Geometry: see drawing. Coordinates: mm, zero at the bounding-box minimum. A direction names the side the tool comes from. Coordinates: 2 decimals unless noted, no trailing zeros. Write each loop counter-clockwise with the first axis right and the second up, starting at its lowest first coordinate (ties: lowest second). Pieces come first, ordered by that corner, then holes. Notation, with made-up numbers: (54, 87.5) - (70, 87.5) arc R21 cw to (70, 113.5) - close; hole circle Ø11 at (-6, -20.75). An arc over 180 degrees is marked (long way). One line per question, with ' | ' between items. Start each with the question number.
1) Draft query along Y for the marked faces 1, 2 and 3. Return one class per face: released by +Y, released by -Y, zero draft, split by the parting line, or undercut.
2) Line query: line 1 (Z direction, x = 16.2, y = 26.2); line 2 (Y direction, x = 9.35, z = 1.75); line 3 (Z direction, x = 17.75, y = 1.75). Output: solid intervals per line, ascending.
3) Section query D-D on z = 8. Return loops of the section in (x, y), and give its area (3 significant figures).
4) Section query A-A on y = 14.35. Return loops of the section in (x, z), and give its area (3 significant figures).
5) First-contact query: P1, Ø8, axis at x = 9.35, y = 14.35, coming from the +Z side. Flat tip, straight axial feed; report the tip coordinate or a pass-through.
6) Section query B-B on z = 0.75. Return loops of the section in (x, y), and give its area (3 significant figures).
7) Reachability of the marked faces 4 and 5 from +Z, -Z, +X, -X, +Y, -Y: full face, straight path, thin tool, end or side. Return the list, or none.
8) Section query C-C on x = 17.5. Return loops of the section in (y, z), and give its area (3 significant figures).
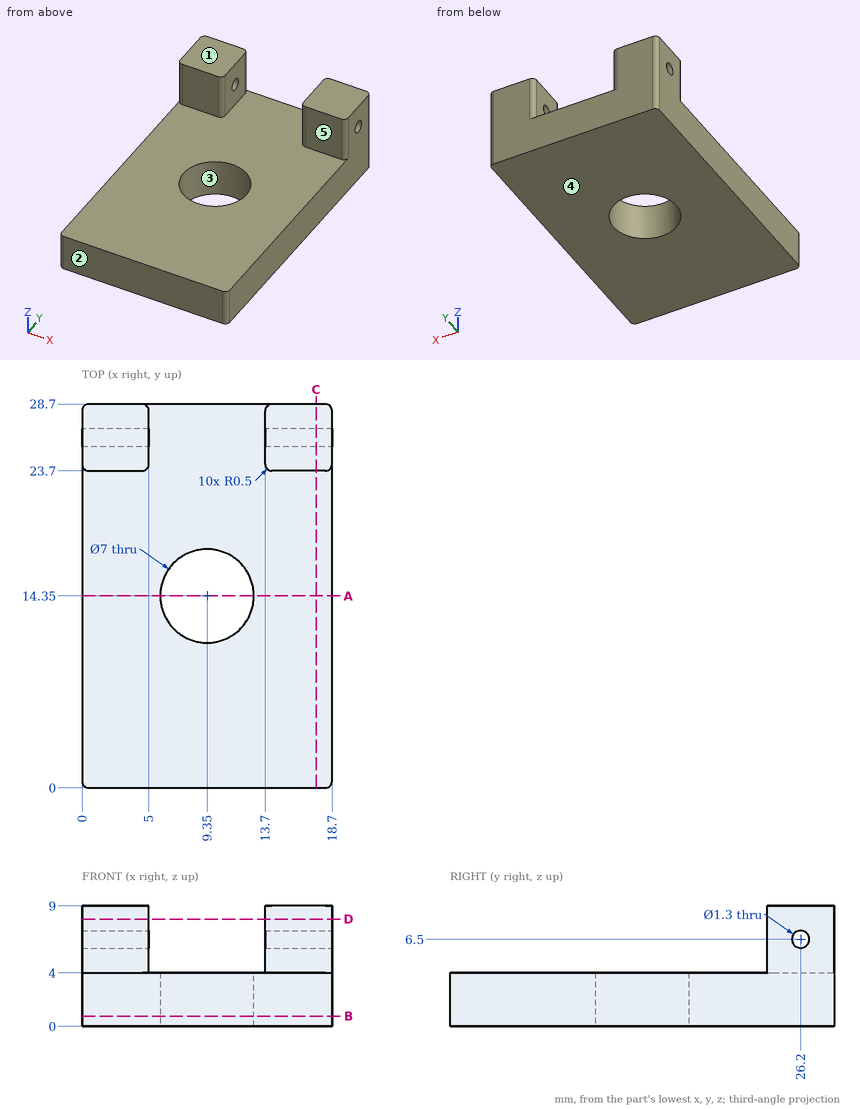
Answer key:
1) face 1: zero draft | face 2: released by -Y | face 3: undercut
2) line 1: 0 to 5.85, 7.15 to 9 | line 2: 0 to 10.85, 17.85 to 28.7 | line 3: 0 to 4
3) outline: (0, 24.2) arc R0.5 ccw to (0.5, 23.7) - (4.5, 23.7) arc R0.5 ccw to (5, 24.2) - (5, 28.2) arc R0.5 ccw to (4.5, 28.7) - (0.5, 28.7) arc R0.5 ccw to (0, 28.2) - close; (13.7, 24.2) arc R0.5 ccw to (14.2, 23.7) - (18.2, 23.7) arc R0.5 ccw to (18.7, 24.2) - (18.7, 28.2) arc R0.5 ccw to (18.2, 28.7) - (14.2, 28.7) arc R0.5 ccw to (13.7, 28.2) - close | area: 49.6 mm²
4) outline: (0, 0) - (5.85, 0) - (5.85, 4) - (0, 4) - close; (12.85, 0) - (18.7, 0) - (18.7, 4) - (12.85, 4) - close | area: 46.8 mm²
5) P1: z = 4
6) outline: (0, 0.5) arc R0.5 ccw to (0.5, 0) - (18.2, 0) arc R0.5 ccw to (18.7, 0.5) - (18.7, 28.2) arc R0.5 ccw to (18.2, 28.7) - (0.5, 28.7) arc R0.5 ccw to (0, 28.2) - close; hole circle Ø7 at (9.35, 14.35) | area: 498 mm²
7) face 4: -Z, +X, -X, +Y, -Y | face 5: +Z, +X, -X, -Y
8) outline: (0, 0) - (28.7, 0) - (28.7, 9) - (23.7, 9) - (23.7, 4) - (0, 4) - close; hole circle Ø1.3 at (26.2, 6.5) | area: 138 mm²
